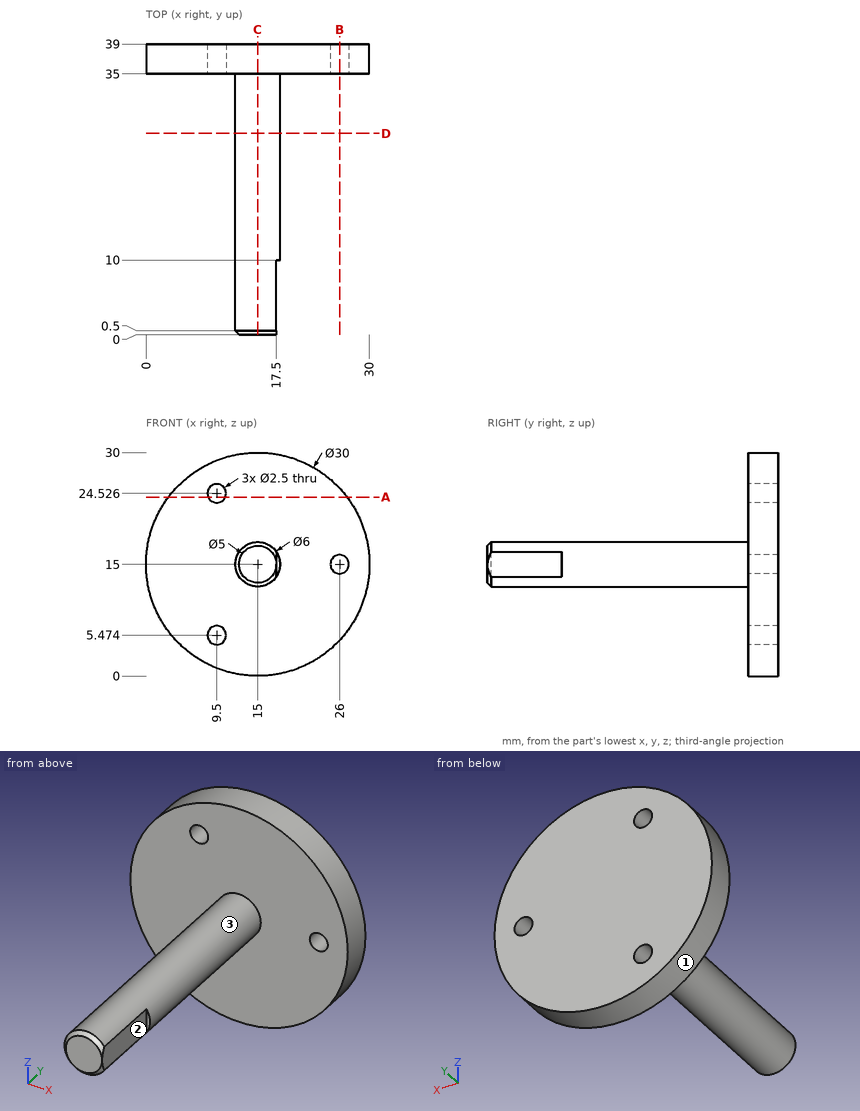
Here's the drawing with two shaded views (mm, measured from the low corner). I have some questions. A direction names the side the tool comes from. Give positions to 0.01 mm unless a question says otherwise; leave off trailing zeros. Loops run counter-clockwise (first coordinate to the right, second up) from the corner with the lowest first, then second, coordinate; pieces in that order, holes last. Notation, with made-up numbers: (60, -23) -> (99, -23) arc R20 cw to (99, 10) -> close; hole circle Ø6 at (-25.5, 75). An arc over 180 degrees is marked (long way). Answer as a JSON object with one key per item and string values. Group by question number.
Item 1: On a 3-axis mill with a long thin cutter (end or side, diameter ignored), from which of +Z, -Z, +X, -X, +Y, -Y can I reach the whole of each face in a straight line? I mean the marked faces 1, 2 and 3. Say none if no direction works.
Item 2: I need wall thicknesses on L1, parallel to Z at x = 9.5, y = 37.3 (1 decimal); L2, parallel to Y at x = 6.75, z = 17.5; L3, parallel to X at y = 14, z = 16.75. Which ranges of each line are inside material? Lowest first, please.
Item 3: Imagine slicing it at B-B on x = 26. Write out the boundary of the cut face in (y, z), then the cut area to 3 significant figures.
Item 4: Imagine slicing it at D-D on y = 27. Write out the boundary of the cut face in (x, z).
Item 5: Will these pins go through, and if not, where does the flat tip stop? pin 1 (1.7 mm diameter, centred on y = 4.5, z = 14.5, fed in from +X); pin 2 (10 mm diameter, centred on x = 22, y = 7.5, fed in from +Z); pin 3 (1 mm diameter, centred on x = 15.5, y = 24.5, fed in from -Z).
Item 6: Imagine slicing it at A-A on z = 24. Write out the boundary of the cut face in (x, y).
Item 7: Imagine slicing it at C-C on x = 15. Write out the boundary of the cut face in (y, z).
Answer list:
{
 "1": {"face 1": "+Y, -Y", "face 2": "+Z, -Z, +X, -Y", "face 3": "-Y"},
 "2": {"L1": "z = 1 to 4.2, 6.7 to 23.3, 25.8 to 29", "L2": "y = 35 to 39", "L3": "x = 12.56 to 17.44"},
 "3": {"outline": "(35, 4.8) -> (39, 4.8) -> (39, 13.75) -> (35, 13.75) -> close; (35, 16.25) -> (39, 16.25) -> (39, 25.2) -> (35, 25.2) -> close", "area": "71.6 mm2"},
 "4": {"outline": "circle Ø6 at (15, 15)"},
 "5": {"pin 1": "stops at x = 17.5", "pin 2": "stops at z = 17.24", "pin 3": "stops at z = 12"},
 "6": {"outline": "(3, 35) -> (8.37, 35) -> (8.37, 39) -> (3, 39) -> close; (10.63, 35) -> (27, 35) -> (27, 39) -> (10.63, 39) -> close"},
 "7": {"outline": "(0, 12.5) -> (0.5, 12) -> (35, 12) -> (35, 0) -> (39, 0) -> (39, 30) -> (35, 30) -> (35, 18) -> (0.5, 18) -> (0, 17.5) -> close"}
}
